Geometry: final body of the model. Coordinates: model frame, mm. Round coordinates to 2 decimals unless told otherwise and drop trailing zeros. Loops run counter-clockwise (first coordinate to the right, second up) from the corner with the lowest first, then second, coordinate; pieces in that order, holes last. Notation, with made-up numbers: (11, 89) - (35, 89) arc R19 ccw to (35, 107) - close; hole circle Ø7 at (41, 73.5). An arc over 180 degrees is marked (long way). Use CSV: the item, a comma, the result in double quotes.
from build123d import *

# Parameters (mm, degrees)
F0_R      = 20.6375
F1_DEPTH  = 23.8252
F3_D      = 15.875
F3_DEPTH  = 12.7
F5_D      = 15.875
F5_DEPTH  = 12.7
F7_D      = 15.875
F7_DEPTH  = 12.7
F9_D      = 15.875
F9_DEPTH  = 12.7
F11_D     = 15.875
F11_DEPTH = 12.7


with BuildPart() as f1:
    # F0 (on Front) → F1 (new body)
    with BuildSketch(Plane.XZ):
        Polygon((-7.358128, 32.536745), (-33.21807, 3.056411), (-13.171768, -30.647779), (25.07747, -21.99778), (28.670496, 17.052403), align=None)
        Circle(F0_R, mode=Mode.SUBTRACT)
    extrude(amount=F1_DEPTH)

    # F3
    with Locations(Plane(origin=(26.873983, 0, -2.472689), x_dir=(0, 1, 0), z_dir=(0.995794, 0, -0.091623))):
        with Locations((-11.9126, 0)):
            Hole(F3_D / 2, depth=F3_DEPTH)

    # F5
    with Locations(Plane(origin=(10.656184, 0, 24.794574), x_dir=(0.918743, 0, -0.394856), z_dir=(0.394856, 0, 0.918743))):
        with Locations((0, -11.9126)):
            Hole(F5_D / 2, depth=F5_DEPTH)

    # F7
    with Locations(Plane(origin=(-23.194919, 0, -13.795684), x_dir=(0, -1, 0), z_dir=(-0.859469, 0, -0.511188))):
        with Locations((11.9126, 0)):
            Hole(F7_D / 2, depth=F7_DEPTH)

    # F9
    with Locations(Plane(origin=(-20.288099, 0, 17.796578), x_dir=(0, -1, 0), z_dir=(-0.751759, 0, 0.659438))):
        with Locations((11.9126, 0)):
            Hole(F9_D / 2, depth=F9_DEPTH)

    # F11
    with Locations(Plane(origin=(5.952851, 0, -26.32278), x_dir=(0.975369, 0, 0.220578), z_dir=(0.220578, 0, -0.975369))):
        with Locations((0, 11.9126)):
            Hole(F11_D / 2, depth=F11_DEPTH)


solid = f1.part
Item 1: Section A-A on x = -6.5. Return the cut outline in (y, z), plus the area to 3 significant figures.
Final values:
outline,"(-23.83, -29.14) - (0, -29.14) - (0, -19.59) - (-23.83, -19.59) - close; (-23.83, 19.59) - (0, 19.59) - (0, 32.17) - (-23.83, 32.17) - close"
area,"527 mm²"
Item 2: Mould query, pull axis X, two halves, no side actions, for faces 1 (the cylindrical face through (22.42, -5.61, -6.91)), 2 (the flat face through (18, -23.825, -11)), 3 (the flat face through (-23.335, -3.804, -13.56)). Classes: released by +X, released by -X, zero draft, split by the parting line, or undercut.
Final values:
face 1,"undercut"
face 2,"zero draft"
face 3,"released by -X"
Item 3: Section B-B on y = -7. Return the cut outline in (x, z) (1 decimal), plus the area to 3 significant figures.
Final values:
outline,"(-33.2, 3.1) - (-26.4, -8.4) - (-20.1, -4.7) arc R20.6 cw to (-18.9, 8.3) - (-24.4, 13.1) - close; (-20, -19.2) - (-13.2, -30.6) - (-0.1, -27.7) - (-1.7, -20.6) arc R20.6 cw to (-13.7, -15.4) - close; (-16.2, 22.5) - (-10.7, 17.7) arc R20.6 cw to (2, 20.5) - (4.9, 27.3) - (-7.4, 32.5) - close; (10.4, -17.8) - (12, -24.9) - (25.1, -22) - (26.3, -8.7) - (19, -8) arc R20.6 cw to start; (13.5, 15.6) arc R20.6 cw to (20.2, 4.4) - (27.4, 3.7) - (28.7, 17.1) - (16.4, 22.3) - close"
area,"892 mm²"
Item 4: Section C-C on y = -21.5. Return the cut outline in (x, z) (1 decimal), plus the area to 3 significant figures.
Final values:
outline,"(-33.2, 3.1) - (-13.2, -30.6) - (25.1, -22) - (28.7, 17.1) - (-7.4, 32.5) - close; hole circle Ø41.3 at (0, 0)"
area,"1,310 mm²"
Item 5: Material intervals for line 1 (Z direction, x = -3.5, y = -19); line 2 (Y direction, x = -19.5, z = 18); line 3 (Z direction, x = -6, y = -13.75), sorted ascending.
Final values:
line 1,"z = -28.46 to -20.34, 20.34 to 30.88"
line 2,"y = -23.83 to -19.82, -4 to 0"
line 3,"z = -29.03 to -19.75, 19.75 to 31.95"
Item 6: Section D-D on z = 16. Give the number of separate pieces and of enclosed holes in the cut face, plus the area to 3 significant figures.
Final values:
separate pieces,"3"
enclosed holes,"0"
area,"425 mm²"
Item 7: Pin query (flat end, axial travel): P1, Ø2, axis at x = -22, y = -10.5, coming from the -Z side; P2, Ø5, axis at y = -18, z = -19.5, coming from the +X side; P3, Ø2, axis at x = -23, y = -9, coming from the +Z side. Return the tip coordinate at first contact, or that it passes through.
Final values:
P1,"stops at z = -4.64"
P2,"stops at x = 25.54"
P3,"stops at z = 11.41"
